from build123d import *

# Parameters (mm, degrees)
SKETCH1_W           = 220
SKETCH1_H           = 175
BOSS_EXTRUDE1_DEPTH = 5
SKETCH2_W           = 15
SKETCH2_H           = 5
CUT_EXTRUDE1_DEPTH  = 282.15831839
LPATTERN1_COUNT     = 7
LPATTERN1_PITCH     = 30
SKETCH3_W           = 15
SKETCH3_H           = 5.956499639
CUT_EXTRUDE2_DEPTH  = 282.15831839
LPATTERN2_COUNT     = 7
LPATTERN2_PITCH     = 30
SKETCH4_R           = 1.5
CUT_EXTRUDE3_DEPTH  = 282.15831839
SKETCH5_W           = 5
SKETCH5_H           = 15
CUT_EXTRUDE4_DEPTH  = 282.15831839
SKETCH7_W           = 40
SKETCH7_H           = 44.8382835
SKETCH7_W_2         = 10
SKETCH7_H_2         = 7.632708493
CUT_EXTRUDE6_DEPTH  = 282.15831839
SKETCH8_W           = 5
SKETCH8_H           = 10
CUT_EXTRUDE7_DEPTH  = 282.15831839
CUT_EXTRUDE8_DEPTH  = 282.15831839


with BuildPart() as part:
    # Sketch1 → Boss-Extrude1 (new body)
    with BuildSketch(Plane.XY):
        with Locations((-110, 87.5)):
            Rectangle(SKETCH1_W, SKETCH1_H)
    extrude(amount=BOSS_EXTRUDE1_DEPTH)

    # Sketch2 → Cut-Extrude1 (cut, through all)
    with BuildSketch(Plane.XY.offset(5)):
        with Locations((-197.5, 2.5)):
            Rectangle(SKETCH2_W, SKETCH2_H)
    cut_extrude1 = extrude(amount=-CUT_EXTRUDE1_DEPTH, mode=Mode.SUBTRACT)

    # LPattern1: Cut-Extrude1 ×7
    with Locations(*[(i * LPATTERN1_PITCH, 0, 0) for i in range(1, LPATTERN1_COUNT)]):
        add(cut_extrude1, mode=Mode.SUBTRACT)

    # Sketch3 → Cut-Extrude2 (cut, through all)
    with BuildSketch(Plane.XY.offset(5)):
        with Locations((-197.5, 172.021750181)):
            Rectangle(SKETCH3_W, SKETCH3_H)
    cut_extrude2 = extrude(amount=-CUT_EXTRUDE2_DEPTH, mode=Mode.SUBTRACT)

    # LPattern2: Cut-Extrude2 ×7
    with Locations(*[(i * LPATTERN2_PITCH, 0, 0) for i in range(1, LPATTERN2_COUNT)]):
        add(cut_extrude2, mode=Mode.SUBTRACT)

    # Sketch4 → Cut-Extrude3 (cut, through all)
    with BuildSketch(Plane.XY.offset(5)):
        with Locations((-12, 15)):
            Circle(SKETCH4_R)
    extrude(amount=-CUT_EXTRUDE3_DEPTH, mode=Mode.SUBTRACT)

    # Sketch5 → Cut-Extrude4 (cut, through all)
    with BuildSketch(Plane(origin=(0, 0, 0), x_dir=(-1, 0, 0), z_dir=(0, 0, -1))):
        with Locations((2.5, 107.048065362)):
            Rectangle(SKETCH5_W, SKETCH5_H)
        with Locations((2.5, 12.048065362)):
            Rectangle(SKETCH5_W, SKETCH5_H)
    extrude(amount=-CUT_EXTRUDE4_DEPTH, mode=Mode.SUBTRACT)

    # Sketch7 → Cut-Extrude6 (cut, through all)
    with BuildSketch(Plane.XY.offset(5)):
        with Locations((-20, 152.58085825)):
            Rectangle(SKETCH7_W, SKETCH7_H)
        with Locations((-50, 133.978070747)):
            Rectangle(SKETCH7_W_2, SKETCH7_H_2)
    extrude(amount=-CUT_EXTRUDE6_DEPTH, mode=Mode.SUBTRACT)

    # Sketch8 → Cut-Extrude7 (cut, through all)
    with BuildSketch(Plane.XY.offset(5)):
        with BuildLine():
            Line((-220, 175), (-65, 175))
            Line((-65, 175), (-65, 45))
            ThreePointArc((-65, 45), (-67.928932188, 37.928932188), (-75, 35))
            Line((-75, 35), (-210, 35))
            ThreePointArc((-210, 35), (-217.071067812, 32.071067812), (-220, 25))
            Line((-220, 25), (-220, 175))
        make_face()
        with Locations((-197.5, 18.629836595)):
            Rectangle(SKETCH8_W, SKETCH8_H)
        with Locations((-112.5, 18.629836595)):
            Rectangle(SKETCH8_W, SKETCH8_H)
    extrude(amount=-CUT_EXTRUDE7_DEPTH, mode=Mode.SUBTRACT)

    # Sketch9 → Cut-Extrude8 (cut, through all)
    with BuildSketch(Plane.XY.offset(5)):
        with BuildLine():
            Line((-214, 11), (-211, 11))
            ThreePointArc((-211, 11), (-210, 10), (-211, 9))
            Line((-211, 9), (-214, 9))
            ThreePointArc((-214, 9), (-215, 10), (-214, 11))
        make_face()
        with BuildLine():
            Line((-154, 11), (-151, 11))
            ThreePointArc((-151, 11), (-150, 10), (-151, 9))
            Line((-151, 9), (-154, 9))
            ThreePointArc((-154, 9), (-155, 10), (-154, 11))
        make_face()
        with BuildLine():
            Line((-94, 11), (-91, 11))
            ThreePointArc((-91, 11), (-90, 10), (-91, 9))
            Line((-91, 9), (-94, 9))
            ThreePointArc((-94, 9), (-95, 10), (-94, 11))
        make_face()
        with BuildLine():
            Line((-34, 11), (-31, 11))
            ThreePointArc((-31, 11), (-30, 10), (-31, 9))
            Line((-31, 9), (-34, 9))
            ThreePointArc((-34, 9), (-35, 10), (-34, 11))
        make_face()
        with BuildLine():
            Line((-11, 30), (-11, 33))
            ThreePointArc((-11, 33), (-10, 34), (-9, 33))
            Line((-9, 33), (-9, 30))
            ThreePointArc((-9, 30), (-10, 29), (-11, 30))
        make_face()
        with BuildLine():
            Line((-11, 107.1617165), (-11, 110.1617165))
            ThreePointArc((-11, 110.1617165), (-10, 111.1617165), (-9, 110.1617165))
            Line((-9, 110.1617165), (-9, 107.1617165))
            ThreePointArc((-9, 107.1617165), (-10, 106.1617165), (-11, 107.1617165))
        make_face()
        with BuildLine():
            Line((-51.5, 142.794424993), (-48.5, 142.794424993))
            ThreePointArc((-48.5, 142.794424993), (-47.5, 141.794424993), (-48.5, 140.794424993))
            Line((-48.5, 140.794424993), (-51.5, 140.794424993))
            ThreePointArc((-51.5, 140.794424993), (-52.5, 141.794424993), (-51.5, 142.794424993))
        make_face()
        with BuildLine():
            Line((-49.5, 165), (-46.5, 165))
            ThreePointArc((-46.5, 165), (-45.5, 164), (-46.5, 163))
            Line((-46.5, 163), (-49.5, 163))
            ThreePointArc((-49.5, 163), (-50.5, 164), (-49.5, 165))
        make_face()
        with BuildLine():
            Line((-51.5, 134.1617165), (-48.5, 134.1617165))
            ThreePointArc((-48.5, 134.1617165), (-47.5, 133.1617165), (-48.5, 132.1617165))
            Line((-48.5, 132.1617165), (-51.5, 132.1617165))
            ThreePointArc((-51.5, 132.1617165), (-52.5, 133.1617165), (-51.5, 134.1617165))
        make_face()
    extrude(amount=-CUT_EXTRUDE8_DEPTH, mode=Mode.SUBTRACT)


solid = part.part
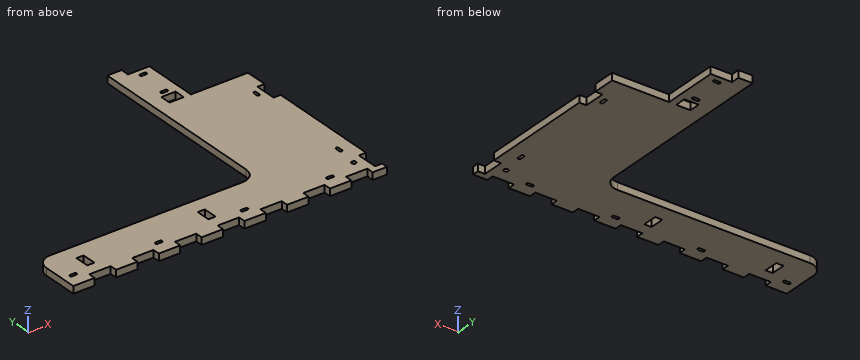
Input: part model. Units: mm. Frame: model coordinates. Round coordinates to 2 decimals unless told otherwise and drop trailing zeros. Write each loop counter-clockwise with the first axis right and the second up, starting at its lowest first coordinate (ties: lowest second). Pieces come first, ordered by that corner, then holes.
1) Ray query, L1, parallel to X at y = 18, z = 3.35; L2, parallel to Y at x = -12, z = 1.45; L3, parallel to Y at x = -154, z = 3.4. Return the intervals inside material, ascending.
2) Cut plane B-B (z = 1.55). Count the separate pieces of the cut face and the enclosed holes in it, then the cut area to 3 significant figures.
3) Cut plane C-C (x = -170.5). Return the cut outline in (y, z).
4) Contact query for flat-ended pins moving along their axis: P1, Ø3, axis at x = -104, z = 4, coming from the +Y side; P2, Ø0.9, axis at y = 31.5, z = 2, coming from the -X side; P3, Ø1.5, axis at y = 108, z = 2.5, coming from the +X side. Output: stop coordinate, or through.
5) Cut plane A-A (y = 133). Return the cut outline in (x, z), then the cut area to 3 significant figures.
Geometry says:
1. L1: x = -220 to -200, -195 to -115, -110 to -5
1. L2: y = 5 to 13.5, 16.5 to 130.16
1. L3: y = 0 to 9, 11 to 35
2. separate pieces: 1
2. enclosed holes: 12
2. area: 14,000 mm2
3. outline: (5, 0) - (35, 0) - (35, 5) - (5, 5) - close
4. P1: stops at y = 35
4. P2: stops at x = -217.96
4. P3: stops at x = -5
5. outline: (-65, 0) - (-55, 0) - (-55, 5) - (-65, 5) - close; (-45, 0) - (-40, 0) - (-40, 5) - (-45, 5) - close
5. area: 75.0 mm2
